from build123d import *

# Parameters (mm, degrees)
BOSS_EXTRUDE1_DEPTH = 5
SKETCH3_R           = 1.25
CUT_EXTRUDE1_DEPTH  = 10


with BuildPart() as part:
    # Sketch2 → Boss-Extrude1 (new body)
    with BuildSketch(Plane.XY):
        with BuildLine():
            ThreePointArc((-8, 0), (0, 8), (8, 0))
            Line((8, 0), (13.6, 0))
            Line((13.6, 0), (13.6, 10))
            Line((13.6, 10), (8.008871246, 10))
            ThreePointArc((8.008871246, 10), (6.357463889, 8.822466805), (4.337930538, 9.01012534))
            ThreePointArc((4.337930538, 9.01012534), (0.001186479, 9.99999993), (-4.335792351, 9.011154459))
            ThreePointArc((-4.335792351, 9.011154459), (-6.353531515, 8.82385013), (-8.003690819, 10))
            Line((-8.003690819, 10), (-13.6, 10))
            Line((-13.6, 10), (-13.6, 0))
            Line((-13.6, 0), (-8, 0))
        make_face()
    extrude(amount=BOSS_EXTRUDE1_DEPTH)

    # Sketch3 → Cut-Extrude1 (cut)
    with BuildSketch(Plane(origin=(0, 10, 0), x_dir=(1, 0, 0), z_dir=(0, 1, 0))):
        with Locations(Location((-10.998930891, -2.5, 0), (0, 0, 270))):
            Circle(SKETCH3_R)
        with Locations(Location((11.001069109, -2.5, 0), (0, 0, 270))):
            Circle(SKETCH3_R)
    extrude(amount=-CUT_EXTRUDE1_DEPTH, mode=Mode.SUBTRACT)


solid = part.part
Source: CAD feature listing. Evaluate the final solid. Frame: model axes, mm. Round coordinates to 2 decimals unless told otherwise and drop trailing zeros. Loops run counter-clockwise (first coordinate to the right, second up) from the corner with the lowest first, then second, coordinate; pieces in that order, holes last. Notation, with made-up numbers: (-38.75, 23) - (-3.75, 23) arc R10 ccw to (-3.75, 32) - close; hole circle Ø2 at (32, 61.5). An arc over 180 degrees is marked (long way). Write item = value, one per line. Start each with the question number.
Item 1: Material intervals for line 1 (X direction, y = 5.75, z = 2.5); line 2 (X direction, y = 3, z = 2.5); line 3 (X direction, y = 6.75, z = 0.45), sorted ascending.
Item 2: Section query D-D on x = 0. Output: boundary loops of the cut face in (y, z).
Item 3: Mould query, pull axis Z, two halves, no side actions, for faces 1 (the face through (-9.59, 0, 2.46)), 2 (the face through (-11.478, 5.07, 3.655)), 3 (the face through (-0.2, 8.4, 5)), 4 (the face through (9.892, 5.07, 3.077)). Classes: released by +Z, released by -Z, zero draft, split by the parting line, or undercut.
Item 4: Section query C-C on y = 2.25. Output: boundary loops of the cut face in (x, z), plus the area to 3 significant figures.
Item 5: Section query A-A on y = 5.5. Output: boundary loops of the cut face in (x, z).
Item 6: Section query B-B on z = 3.4. Output: boundary loops of the cut face in (x, y), plus the area to 3 significant figures.
Results list:
q1.line_1 = -13.6 to -12.25, -9.75 to -5.56, 5.56 to 9.75, 12.25 to 13.6
q1.line_2 = -13.6 to -12.25, -9.75 to -7.42, 7.42 to 9.75, 12.25 to 13.6
q1.line_3 = -13.6 to -4.29, 4.29 to 13.6
q2.outline = (8, 0) - (10, 0) - (10, 5) - (8, 5) - close
q3.face_1 = zero draft
q3.face_2 = undercut
q3.face_3 = released by +Z
q3.face_4 = undercut
q4.outline = (-13.6, 0) - (-7.68, 0) - (-7.68, 5) - (-13.6, 5) - close; (7.68, 0) - (13.6, 0) - (13.6, 5) - (7.68, 5) - close; hole circle Ø2.5 at (-11, 2.5); hole circle Ø2.5 at (11, 2.5)
q4.area = 49.4 mm²
q5.outline = (-13.6, 0) - (-5.81, 0) - (-5.81, 5) - (-13.6, 5) - close; (5.81, 0) - (13.6, 0) - (13.6, 5) - (5.81, 5) - close; hole circle Ø2.5 at (-11, 2.5); hole circle Ø2.5 at (11, 2.5)
q6.outline = (-13.6, 0) - (-11.87, 0) - (-11.87, 10) - (-13.6, 10) - close; (-10.13, 0) - (-8, 0) arc R8 cw to (8, 0) - (10.13, 0) - (10.13, 10) - (8.01, 10) arc R2.91 cw to (4.34, 9.01) arc R10 ccw to (-4.34, 9.01) arc R2.91 cw to (-8, 10) - (-10.13, 10) - close; (11.87, 0) - (13.6, 0) - (13.6, 10) - (11.87, 10) - close
q6.area = 127 mm²
